Read the model definition and answer for the solid it produces. Units are mm, in the model's axes. Round coordinates to 2 decimals unless told otherwise and drop trailing zeros. Order: outer loops, then holes, each group sorted by start corner. A loop starts at its lowest first (then second) coordinate and runs counter-clockwise, first axis right, second up.
from build123d import *

# Parameters (mm, degrees)
SKETCH1_W           = 126.746
SKETCH1_H           = 241.3
BOSS_EXTRUDE1_DEPTH = 2.9972
CUT_EXTRUDE1_DEPTH  = 137.314132931


with BuildPart() as part:
    # Sketch1 → Boss-Extrude1 (new body)
    with BuildSketch(Plane.XY):
        Rectangle(SKETCH1_W, SKETCH1_H)
    extrude(amount=BOSS_EXTRUDE1_DEPTH)

    # Sketch2 → Cut-Extrude1 (cut, through all)
    with BuildSketch(Plane.XY.offset(2.9972)):
        with BuildLine():
            Line((-38.1, -63.375), (38.1, -63.375))
            ThreePointArc((38.1, -63.375), (41.275, -66.55), (38.1, -69.725))
            Line((38.1, -69.725), (-38.1, -69.725))
            ThreePointArc((-38.1, -69.725), (-41.275, -66.55), (-38.1, -63.375))
        make_face()
        with BuildLine():
            Line((-38.1, -84.075), (38.1, -84.075))
            ThreePointArc((38.1, -84.075), (41.275, -87.25), (38.1, -90.425))
            Line((38.1, -90.425), (-38.1, -90.425))
            ThreePointArc((-38.1, -90.425), (-41.275, -87.25), (-38.1, -84.075))
        make_face()
        with BuildLine():
            Line((-38.1, -104.775), (38.1, -104.775))
            ThreePointArc((38.1, -104.775), (41.275, -107.95), (38.1, -111.125))
            Line((38.1, -111.125), (-38.1, -111.125))
            ThreePointArc((-38.1, -111.125), (-41.275, -107.95), (-38.1, -104.775))
        make_face()
        with BuildLine():
            Line((-38.1, -73.725), (38.1, -73.725))
            ThreePointArc((38.1, -73.725), (41.275, -76.9), (38.1, -80.075))
            Line((38.1, -80.075), (-38.1, -80.075))
            ThreePointArc((-38.1, -80.075), (-41.275, -76.9), (-38.1, -73.725))
        make_face()
        with BuildLine():
            Line((-38.1, -94.425), (38.1, -94.425))
            ThreePointArc((38.1, -94.425), (41.275, -97.6), (38.1, -100.775))
            Line((38.1, -100.775), (-38.1, -100.775))
            ThreePointArc((-38.1, -100.775), (-41.275, -97.6), (-38.1, -94.425))
        make_face()
    extrude(amount=-CUT_EXTRUDE1_DEPTH, mode=Mode.SUBTRACT)


solid = part.part
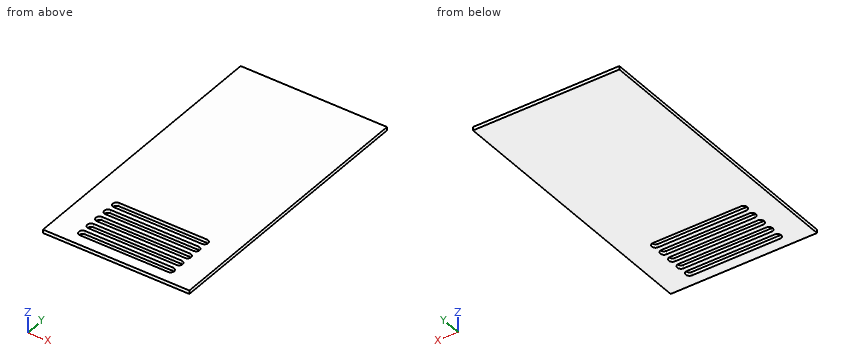
Q1. A flat-ended cylindrical pin translates along its axis: pin 1 (6 mm diameter, centred on x = -17.5, y = -2.5, fed in from -Z). Find the tip coordinate at first contact, or state that the pin passes through.
Outcome:
pin 1: stops at z = 0
Q2. Straight lines are drawn through the part: probe 1 along Y at (x, z) = (31.5, 2.1) (3 decimals); probe 2 along X at (y, z) = (-76, 0.6); probe 3 along X at (y, z) = (-69, 2.5). For each, find the intervals that lie inside material, in ascending order.
Outcome:
probe 1: y = -120.65 to -111.125, -104.775 to -100.775, -94.425 to -90.425, -84.075 to -80.075, -73.725 to -69.725, -63.375 to 120.65
probe 2: x = -63.37 to -41.14, 41.14 to 63.37
probe 3: x = -63.37 to -40.12, 40.12 to 63.37
Q3. A cutting plane is placed at B-B, the plane y = -97.6. Give the vertices of the cut face in (x, z) (3 decimals).
Outcome:
outline: (-63.373, 0) - (-41.275, 0) - (-41.275, 2.997) - (-63.373, 2.997) - close; (41.275, 0) - (63.373, 0) - (63.373, 2.997) - (41.275, 2.997) - close
Q4. A cutting plane is placed at A-A, the plane x = -34. Give the vertices of the cut face in (y, z) (3 decimals), plus the area to 3 significant figures.
Outcome:
outline: (-120.65, 0) - (-111.125, 0) - (-111.125, 2.997) - (-120.65, 2.997) - close; (-104.775, 0) - (-100.775, 0) - (-100.775, 2.997) - (-104.775, 2.997) - close; (-94.425, 0) - (-90.425, 0) - (-90.425, 2.997) - (-94.425, 2.997) - close; (-84.075, 0) - (-80.075, 0) - (-80.075, 2.997) - (-84.075, 2.997) - close; (-73.725, 0) - (-69.725, 0) - (-69.725, 2.997) - (-73.725, 2.997) - close; (-63.375, 0) - (120.65, 0) - (120.65, 2.997) - (-63.375, 2.997) - close
area: 628 mm2
Q5. A cutting plane is placed at C-C, the plane z = 0.95. Give the vertices of the cut face in (x, y) (3 decimals).
Outcome:
outline: (-63.373, -120.65) - (63.373, -120.65) - (63.373, 120.65) - (-63.373, 120.65) - close; hole (-38.1, -111.125) - (38.1, -111.125) arc R3.175 ccw to (38.1, -104.775) - (-38.1, -104.775) arc R3.175 ccw to start; hole (-38.1, -100.775) - (38.1, -100.775) arc R3.175 ccw to (38.1, -94.425) - (-38.1, -94.425) arc R3.175 ccw to start; hole (-38.1, -90.425) - (38.1, -90.425) arc R3.175 ccw to (38.1, -84.075) - (-38.1, -84.075) arc R3.175 ccw to start; hole (-38.1, -80.075) - (38.1, -80.075) arc R3.175 ccw to (38.1, -73.725) - (-38.1, -73.725) arc R3.175 ccw to start; hole (-38.1, -69.725) - (38.1, -69.725) arc R3.175 ccw to (38.1, -63.375) - (-38.1, -63.375) arc R3.175 ccw to start
